Input: part model. Units: mm. Frame: model coordinates. Face numbers are marked on the shaded views. A direction names the side the tool comes from. Give positions to 0.01 mm unless a question says otherwise; leave off trailing zeros. Loops run counter-clockwise (first coordinate to the right, second up) from the corner with the lowest first, then second, coordinate; pieces in that order, holes last. Notation, with made-up numbers: M 44,42.25 L 101,42.25 A35 cw 101,81.25 Z; hole C 10,78 d9. An arc over 180 degrees is marked long. Answer as a JSON object with one key per item and string values. Group by question number.
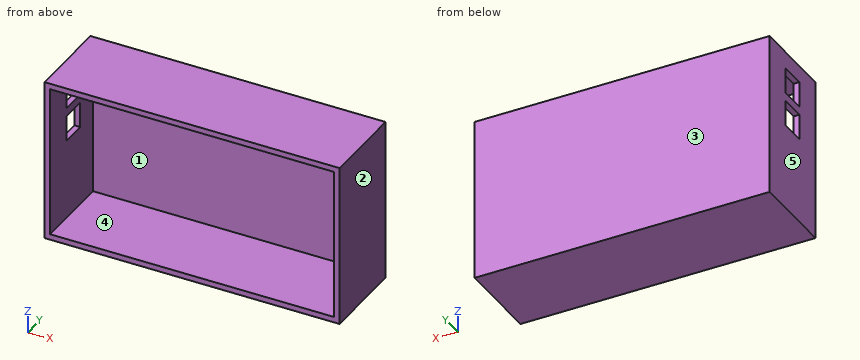
```python
from build123d import *

# Parameters (mm, degrees)
F0_W     = 131.784498
F0_H     = 72.877914
F1_DEPTH = 38.1
F2_T     = -2.54
F3_W     = 11.43
F3_H     = 11.43
F4_DEPTH = 25.4
F5_W     = 11.43
F5_H     = 11.43
F6_DEPTH = 25.4


with BuildPart() as f1:
    # F0 (on Front) → F1 (new body)
    with BuildSketch(Plane.XZ):
        Rectangle(F0_W, F0_H)
    extrude(amount=F1_DEPTH)

    # F2
    f2_openings = [f1.faces().sort_by_distance(p)[0] for p in [
        (0, -38.1, 0),
    ]]
    offset(amount=F2_T, openings=f2_openings)

    # F3 (on face) → F4 (cut)
    with BuildSketch(Plane(origin=(-65.892249, 0, 0), x_dir=(0, -1, 0), z_dir=(-1, 0, 0))):
        with Locations((18.923, 23.103957)):
            Rectangle(F3_W, F3_H)
    extrude(amount=-F4_DEPTH, mode=Mode.SUBTRACT)

    # F5 (on face) → F6 (cut)
    with BuildSketch(Plane(origin=(-65.892249, 0, 0), x_dir=(0, -1, 0), z_dir=(-1, 0, 0))):
        with Locations((18.923, 7.863193)):
            Rectangle(F5_W, F5_H)
    extrude(amount=-F6_DEPTH, mode=Mode.SUBTRACT)


solid = f1.part
```
1. Section A-A (z = 27). Output: boundary loops of the cut face in (x, y).
2. Section D-D (x = -57). Output: boundary loops of the cut face in (y, z).
3. Section C-C (y = -18.5). Output: boundary loops of the cut face in (x, z), then the cut area to 3 significant figures.
4. Section B-B (y = -28). Output: boundary loops of the cut face in (x, z).
5. Reachability of the marked faces 4 and 5 from +Z, -Z, +X, -X, +Y, -Y: full face, straight path, thin tool, end or side. Return the list, or none.
6. Mould query, pull axis X, two halves, no side actions, for the marked faces 1, 2 and 3. Classes: pulls with the +X half, pulls with the -X half, needs draft (parallel to the pull), parting line crosses it, or undercut.
7. Material intervals for L1, parallel to Z at x = 34, y = -7; L2, parallel to X at y = -23, z = 1.5; L3, parallel to Y at x = -25, z = -30, sorted ascending.
8. First-contact query: P1, Ø1, axis at x = 39.5, z = 3.5, coming from the -Y side; P2, Ø4, axis at x = 10.5, z = 26.5, coming from the +Y side. Flat tips, straight axial feed; report the tip coordinate or a pass-through.
Geometry results:
{
 "1": {"outline": "M -65.89,-38.1 L -63.35,-38.1 L -63.35,-24.64 L -65.89,-24.64 Z; M -65.89,-13.21 L -63.35,-13.21 L -63.35,-2.54 L 63.35,-2.54 L 63.35,-38.1 L 65.89,-38.1 L 65.89,0 L -65.89,0 Z"},
 "2": {"outline": "M -38.1,-36.44 L 0,-36.44 L 0,36.44 L -38.1,36.44 L -38.1,33.9 L -2.54,33.9 L -2.54,-33.9 L -38.1,-33.9 Z"},
 "3": {"outline": "M -65.89,-36.44 L 65.89,-36.44 L 65.89,36.44 L -65.89,36.44 L -65.89,28.82 L -63.35,28.82 L -63.35,33.9 L 63.35,33.9 L 63.35,-33.9 L -63.35,-33.9 L -63.35,2.15 L -65.89,2.15 Z; M -65.89,13.58 L -63.35,13.58 L -63.35,17.39 L -65.89,17.39 Z", "area": "956 mm2"},
 "4": {"outline": "M -65.89,-36.44 L 65.89,-36.44 L 65.89,36.44 L -65.89,36.44 Z; hole M -63.35,-33.9 L 63.35,-33.9 L 63.35,33.9 L -63.35,33.9 Z"},
 "5": {"face 4": "-Y", "face 5": "+Z, -Z, -X, +Y, -Y"},
 "6": {"face 1": "undercut", "face 2": "pulls with the +X half", "face 3": "needs draft"},
 "7": {"L1": "-36.44 to -33.9, 33.9 to 36.44", "L2": "-65.89 to -63.35, 63.35 to 65.89", "L3": "-2.54 to 0"},
 "8": {"P1": "y = -2.54", "P2": "y = 0"}
}
